Build history of the part. All positions in model axes, mm. Give positions to 0.01 mm unless a question says otherwise; leave off trailing zeros. Write each loop counter-clockwise with the first axis right and the second up, starting at its lowest first coordinate (ties: lowest second). Pieces come first, ordered by that corner, then holes.
from build123d import *

# Parameters (mm, degrees)
SKETCH_1_R          = 4.3
SKETCH_1_R_2        = 1.6
EXTRUDE_1_DEPTH     = 4.5
SKETCH_2_R          = 5.1
CUT_EXTRUDE_1_DEPTH = 4


with BuildPart() as part:
    # 草图1 → 凸台-拉伸1 (new body)
    with BuildSketch(Plane(origin=(0, 0, 0), x_dir=(0, 0, -1), z_dir=(1, 0, 0))):
        with BuildLine():
            Line((-61.910667188, -17.784854846), (-10.410879829, -17.636861799))
            ThreePointArc((-10.410879829, -17.636861799), (-6.80853031, -16.954371319), (-3.69429735, -15.01936011))
            Line((-3.69429735, -15.01936011), (6.053738335, -6.112622142))
            ThreePointArc((6.053738335, -6.112622142), (7.885847556, 3.160295303), (0.014361881, 8.393204188))
            Line((0.014361881, 8.393204188), (-61.985382125, 8.215037801))
            Line((-61.985382125, 8.215037801), (-61.910667188, -17.784854846))
        make_face()
        with Locations((0.038787918, -0.106760716)):
            Circle(SKETCH_1_R, mode=Mode.SUBTRACT)
        with Locations((-57.973904035, 4.226548923)):
            Circle(SKETCH_1_R_2, mode=Mode.SUBTRACT)
        with Locations((-29.92229392, -13.692914517)):
            Circle(SKETCH_1_R_2, mode=Mode.SUBTRACT)
        with Locations((-33.97400313, 4.295516556)):
            Circle(SKETCH_1_R_2, mode=Mode.SUBTRACT)
        with Locations((-57.92217831, -13.773376756)):
            Circle(SKETCH_1_R_2, mode=Mode.SUBTRACT)
    extrude(amount=EXTRUDE_1_DEPTH)

    # 草图2 → 切除-拉伸1 (cut)
    with BuildSketch(Plane(origin=(4.5, 0, 0), x_dir=(0, 0, -1), z_dir=(1, 0, 0))):
        with Locations((0.038787918, -0.106760716)):
            Circle(SKETCH_2_R)
    extrude(amount=-CUT_EXTRUDE_1_DEPTH, mode=Mode.SUBTRACT)


solid = part.part
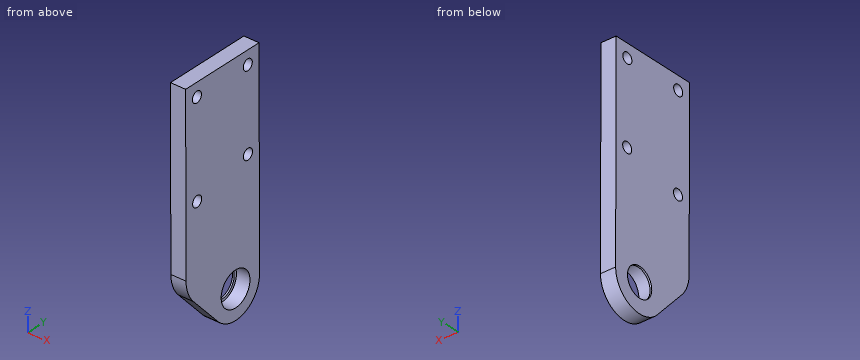
1. Drop flat-ended pins along their axis: pin 1 (1 mm diameter, centred on x = 2, y = 1, fed in from -Z); pin 2 (1.5 mm diameter, centred on x = 1.5, z = 49.5, fed in from -Y); pin 3 (1.5 mm diameter, centred on x = 2.5, y = 0.5, fed in from +Z). Give the stop position or say it passes through.
2. Saw through at A-A on y = -13. Give the cut face in (x, z), plus the area to 3 significant figures.
3. Saw through at B-B on z = 29.5. Give the cut face in (x, y).
4. Drill centre lines: line 1 along Z through (x, y) = (2.6, -14.25); line 2 along Z through (x, y) = (3.1, 5.5); line 3 along Y through (x, z) = (3.8, 33.5). Where is each one in solid material? Low to high.
5. Saw through at C-C on y = -3.75. Give the cut face in (x, z).
6. Saw through at D-D on x = 3.75. Give the cut face in (y, z), plus the area to 3 significant figures.
Outcome:
1. pin 1: stops at z = -8.52
1. pin 2: stops at y = -17.75
1. pin 3: stops at z = 61.97
2. outline: (0, 1.48) - (4.5, 1.48) - (4.5, 28.48) - (0, 28.48) - close; (0, 31.36) - (4.5, 31.36) - (4.5, 56.52) - (0, 56.52) - close; (0, 59.32) - (4.5, 59.32) - (4.5, 61.92) - (0, 61.92) - close
2. area: 246 mm2
3. outline: (0, -17.69) - (4.5, -17.69) - (4.5, -15.24) - (0, -15.24) - close; (0, -12.15) - (4.5, -12.15) - (4.5, 8.31) - (0, 8.31) - close
4. line 1: z = 2.85 to 28.42, 31.42 to 56.39, 59.45 to 61.92
4. line 2: z = -6.43 to 32.92, 35.03 to 57.01, 58.94 to 61.98
4. line 3: y = -17.7 to 2.77, 5.82 to 8.3
5. outline: (0, -7.72) - (4.5, -7.72) - (4.5, -3.61) - (0.5, -3.61) - (0.5, -2.32) - (0, -2.32) - close; (0, 2.25) - (0.5, 2.25) - (0.5, 3.53) - (4.5, 3.53) - (4.5, 61.95) - (0, 61.95) - close
6. outline: (-17.78, 61.91) - (-17.64, 10.41) arc R10 ccw to (-15.02, 3.69) - (-6.11, -6.05) arc R8.5 ccw to (8.39, -0.01) - (8.22, 61.99) - close; hole circle Ø3.2 at (-13.77, 57.92); hole circle Ø3.2 at (-13.69, 29.92); hole circle Ø10.2 at (-0.11, -0.04); hole circle Ø3.2 at (4.23, 57.97); hole circle Ø3.2 at (4.3, 33.97)
6. area: 1,600 mm2
